```python
from build123d import *

# Parameters (mm, degrees)
BOSS_EXTRUDE1_DEPTH = 2
SKETCH2_W           = 18.8
SKETCH2_H           = 15.2
SKETCH2_W_2         = 15.8
SKETCH2_H_2         = 15.8
CUT_EXTRUDE1_DEPTH  = 1.4
SKETCH3_W           = 16.8
SKETCH3_H           = 13.2
SKETCH3_W_2         = 13.8
SKETCH3_H_2         = 13.8
CUT_EXTRUDE2_DEPTH  = 25.191114071
BOSS_EXTRUDE3_DEPTH = 12
FILLET1_R           = 10
SKETCH15_W          = 38
SKETCH15_H          = 16.8
CUT_EXTRUDE3_DEPTH  = 27.96757312
CUT_EXTRUDE5_REACH  = 35.797
SKETCH17_R          = 1


with BuildPart() as part:
    # Sketch1 → Boss-Extrude1 (new body)
    with BuildSketch(Plane(origin=(0, 0, 0), x_dir=(1, 0, 0), z_dir=(0, 1, 0))):
        with BuildLine():
            Line((19.5, -11), (-19.5, -11))
            ThreePointArc((-19.5, -11), (-20.914213562, -10.414213562), (-21.5, -9))
            Line((-21.5, -9), (-21.5, 9))
            ThreePointArc((-21.5, 9), (-20.914213562, 10.414213562), (-19.5, 11))
            Line((-19.5, 11), (19.5, 11))
            ThreePointArc((19.5, 11), (20.914213562, 10.414213562), (21.5, 9))
            Line((21.5, 9), (21.5, -9))
            ThreePointArc((21.5, -9), (20.914213562, -10.414213562), (19.5, -11))
        make_face()
    extrude(amount=BOSS_EXTRUDE1_DEPTH)

    # Sketch2 → Cut-Extrude1 (cut)
    with BuildSketch(Plane(origin=(0, 2, 0), x_dir=(1, 0, 0), z_dir=(0, 1, 0))):
        with Locations((-8.4, -0.4)):
            Rectangle(SKETCH2_W, SKETCH2_H)
        with Locations((9.9, -0.1)):
            Rectangle(SKETCH2_W_2, SKETCH2_H_2)
    extrude(amount=-CUT_EXTRUDE1_DEPTH, mode=Mode.SUBTRACT)

    # Sketch3 → Cut-Extrude2 (cut, through all)
    with BuildSketch(Plane(origin=(0, 0.6, 0), x_dir=(1, 0, 0), z_dir=(0, 1, 0))):
        with Locations((-8.4, -0.4)):
            Rectangle(SKETCH3_W, SKETCH3_H)
        with Locations((9.9, -0.1)):
            Rectangle(SKETCH3_W_2, SKETCH3_H_2)
    extrude(amount=-CUT_EXTRUDE2_DEPTH, mode=Mode.SUBTRACT)

    # Sketch13 → Boss-Extrude3 (add)
    with BuildSketch(Plane(origin=(0, 2, 0), x_dir=(1, 0, 0), z_dir=(0, 1, 0))):
        with BuildLine():
            ThreePointArc((-21.5, -9), (-20.914213562, -10.414213562), (-19.5, -11))
            Line((-19.5, -11), (19.5, -11))
            ThreePointArc((19.5, -11), (20.914213562, -10.414213562), (21.5, -9))
            Line((21.5, -9), (21.5, 9))
            ThreePointArc((21.5, 9), (20.914213562, 10.414213562), (19.5, 11))
            Line((19.5, 11), (-19.5, 11))
            ThreePointArc((-19.5, 11), (-20.914213562, 10.414213562), (-21.5, 9))
            Line((-21.5, 9), (-21.5, -9))
        make_face()
        with BuildLine():
            ThreePointArc((17.5, 8), (18.207106781, 7.707106781), (18.5, 7))
            Line((18.5, 7), (18.5, -7))
            ThreePointArc((18.5, -7), (18.306225775, -7.591607978), (17.8, -7.953939201))
            Line((17.8, -7.953939201), (17.8, -8))
            Line((17.8, -8), (-17.8, -8))
            Line((-17.8, -8), (-17.8, -7.953939201))
            ThreePointArc((-17.8, -7.953939201), (-18.306225775, -7.591607978), (-18.5, -7))
            Line((-18.5, -7), (-18.5, 7))
            ThreePointArc((-18.5, 7), (-18.207106781, 7.707106781), (-17.5, 8))
            Line((-17.5, 8), (17.5, 8))
        make_face(mode=Mode.SUBTRACT)
    extrude(amount=BOSS_EXTRUDE3_DEPTH)

    # Fillet1
    # the kernel refuses this fillet: 10 mm, written as the material it takes off along each edge
    with BuildSketch(Plane(origin=(17.8, 2, 7.953939201), x_dir=(0.906100611464274, 0, -0.42306226717123885), z_dir=(0, 1, 0))) as fillet1_piece_1:
        with BuildLine():
            CenterArc((1.580945974, -9.912835739), FILLET1_R, 97.570469618, 1.638937345)
            Line((-0.019486586, -0.041735718), (0, 0))
            ThreePointArc((0, 0), (0.131745498, -0.008716426), (0.263490996, 0))
        make_face()
    extrude(amount=12.658727489, mode=Mode.SUBTRACT)

    # Sketch15 → Cut-Extrude3 (cut, through all)
    with BuildSketch(Plane(origin=(0, 2, 0), x_dir=(1, 0, 0), z_dir=(0, 1, 0))):
        Rectangle(SKETCH15_W, SKETCH15_H)
    extrude(amount=CUT_EXTRUDE3_DEPTH, mode=Mode.SUBTRACT)

    # Sketch17 → Cut-Extrude5 (cut, up to next)
    with BuildSketch(Plane.XY.offset(11), mode=Mode.PRIVATE) as cut_extrude5_sk1:
        with Locations((0, 7)):
            Circle(SKETCH17_R)
    cut_extrude5_tool1 = extrude(cut_extrude5_sk1.sketch, amount=-CUT_EXTRUDE5_REACH, mode=Mode.PRIVATE) & part.part
    add(cut_extrude5_tool1.solids().sort_by_distance((0, 7, 11))[0], mode=Mode.SUBTRACT)


solid = part.part
```
The model under review builds one solid part; all positions refer to its coordinate system, in mm. A direction names the side the tool comes from. Coordinates: 2 decimals unless noted, no trailing zeros. Write each loop counter-clockwise with the first axis right and the second up, starting at its lowest first coordinate (ties: lowest second). Pieces come first, ordered by that corner, then holes. Notation, with made-up numbers: (45, -40) -> (87, -40) arc R11 ccw to (87, -22) -> close; hole circle Ø1 at (-37.5, 10.25). An arc over 180 degrees is marked (long way). One line per item, written item: value. Start each with the question number.
Q1. Add section D-D, the plane y = 7. Give the boundary of the cut face in (x, z).
Q2. Add section A-A, the plane x = 15. Give the boundary of the cut face in (y, z).
Q3. Add section C-C, the plane y = 2.75. Give the boundary of the cut face in (x, z), then the cut area to 3 significant figures.
Q4. To check wall thickness, follow probe 1 along X at (y, z) = (8.25, 6); probe 2 along Z at (x, y) = (-2, 5.75); probe 3 along Y at (x, z) = (0, 9.75). State the ranges of each line that lie inside material, in increasing order.
Q5. Clearance check with a flat-ended pin moving along its axis: P1, Ø2, axis at x = -8.5, z = -3.5, coming from the +Y side. State where the tip first meets the part, or that it passes through.
Q6. For faces 5 (the face through (0, 8, 10)), 6 (the face through (-19, 8, 0)), 7 (the face through (-21.5, 7, 0)), list the 3-axis set-ups (+Z, -Z, +X, -X, +Y, -Y) from which the entire face can be reached by the end or side of a thin tool; tool diameter is ignored.
Q7. Add section B-B, the plane z = 5.25. Give the boundary of the cut face in (x, y).
Q8. The part is to be moulded in two halves that separate along Z. For faces 1 (the face through (10, 1, -7.8)), 2 (the face through (3, 14, -9)), 3 (the face through (20.9, 6.9, 10.43)), 4 (the face through (-20.9, 6.9, -10.43)), say which applies: +Z half, -Z half, draft (parallel to the pull), parting line (faces both ways), or undercut.
Response:
1. outline: (-21.5, -9) arc R2 ccw to (-19.5, -11) -> (19.5, -11) arc R2 ccw to (21.5, -9) -> (21.5, 9) arc R2 ccw to (19.5, 11) -> (1, 11) -> (1, 8.4) -> (19, 8.4) -> (19, -8.4) -> (-19, -8.4) -> (-19, 8.4) -> (-1, 8.4) -> (-1, 11) -> (-19.5, 11) arc R2 ccw to (-21.5, 9) -> close
2. outline: (0, -11) -> (14, -11) -> (14, -8.4) -> (2, -8.4) -> (2, -7.8) -> (0.6, -7.8) -> (0.6, -6.8) -> (0, -6.8) -> close; (0, 7) -> (0.6, 7) -> (0.6, 8) -> (2, 8) -> (2, 8.4) -> (14, 8.4) -> (14, 11) -> (0, 11) -> close
3. outline: (-21.5, -9) arc R2 ccw to (-19.5, -11) -> (19.5, -11) arc R2 ccw to (21.5, -9) -> (21.5, 9) arc R2 ccw to (19.5, 11) -> (-19.5, 11) arc R2 ccw to (-21.5, 9) -> close; hole (-19, -8.4) -> (19, -8.4) -> (19, 8.4) -> (-19, 8.4) -> close
3. area: 304 mm²
4. probe 1: -21.5 to -19, 19 to 21.5
4. probe 2: -11 to -8.4, 8.4 to 11
4. probe 3: 0 to 6, 8 to 14
5. P1: through
6. face 5: +Z
6. face 6: +Y
6. face 7: +Z, -Z, -X, +Y, -Y
7. outline: (-21.5, 0) -> (-16.8, 0) -> (-16.8, 0.6) -> (-17.8, 0.6) -> (-17.8, 2) -> (-19, 2) -> (-19, 14) -> (-21.5, 14) -> close; (0, 0) -> (3, 0) -> (3, 0.6) -> (2, 0.6) -> (2, 2) -> (1, 2) -> (1, 0.6) -> (0, 0.6) -> close; (16.8, 0) -> (21.5, 0) -> (21.5, 14) -> (19, 14) -> (19, 2) -> (17.8, 2) -> (17.8, 0.6) -> (16.8, 0.6) -> close
8. face 1: undercut
8. face 2: draft
8. face 3: +Z half
8. face 4: -Z half
